```python
from build123d import *

# Parameters (mm, degrees)
BOSS_EXTRUDE1_DEPTH = 7.9
SKETCH2_R           = 1.5
CUT_EXTRUDE1_DEPTH  = 52.15085532
CUT_EXTRUDE3_DEPTH  = 3
BOSS_EXTRUDE2_DEPTH = 3
BOSS_EXTRUDE3_START = -7.9
BOSS_EXTRUDE3_DEPTH = 3
SKETCH5_W           = 8.304797865
SKETCH5_H           = 8.5
CUT_EXTRUDE4_DEPTH  = 49.987855638


with BuildPart() as part:
    # Sketch1 → Boss-Extrude1 (new body)
    with BuildSketch(Plane.XY):
        Polygon((30, 8), (30, 0), (22, 0), (22, -7), (33.5, -7), (45, 4.5), (45, 16), (38, 16), (38, 8), align=None)
    extrude(amount=-BOSS_EXTRUDE1_DEPTH)

    # Sketch2 → Cut-Extrude1 (cut, through all)
    with BuildSketch(Plane.XZ.offset(7)):
        with Locations((27, -3.95)):
            Circle(SKETCH2_R)
    cut_extrude1 = extrude(amount=-CUT_EXTRUDE1_DEPTH, mode=Mode.SUBTRACT)

    # Sketch3 → Cut-Extrude3 (cut)
    with BuildSketch(Plane(origin=(38, -7, 0), x_dir=(0, 0, -1), z_dir=(0, 1, 0))):
        Polygon((0.95, 12.732050808), (3.95, 14.464101615), (6.95, 12.732050808), (6.95, 9.267949192), (3.95, 7.535898385), (0.95, 9.267949192), align=None)
    cut_extrude3 = extrude(amount=CUT_EXTRUDE3_DEPTH, mode=Mode.SUBTRACT)

    # Sketch4 → Boss-Extrude2 (add)
    with BuildSketch(Plane.XY):
        Polygon((22, 0), (38, 16), (45, 16), (45, 4.5), (33.5, -7), (22, -7), align=None)
    extrude(amount=BOSS_EXTRUDE2_DEPTH)

    # Sketch4<3> → Boss-Extrude3 (add)
    with BuildSketch(Plane.XY.offset(BOSS_EXTRUDE3_START)):
        Polygon((30, 8), (22, 0), (30, 0), align=None)
        Polygon((30, 0), (22, 0), (22, -7), (33.5, -7), (45, 4.5), (45, 16), (38, 16), (38, 8), (30, 8), align=None)
        Polygon((38, 16), (30, 8), (38, 8), align=None)
    extrude(amount=-BOSS_EXTRUDE3_DEPTH)

    # Sketch5 → Cut-Extrude4 (cut, through all)
    with BuildSketch(Plane(origin=(0, 0, 0), x_dir=(1, 0, 0), z_dir=(0, 1, 0))):
        with Locations((26.152398932, 3.95)):
            Rectangle(SKETCH5_W, SKETCH5_H)
    cut_extrude4 = extrude(amount=CUT_EXTRUDE4_DEPTH, mode=Mode.SUBTRACT)

    # Mirror1: Cut-Extrude1, Cut-Extrude3, Cut-Extrude4 across plane
    add(cut_extrude1.mirror(Plane(origin=(19, 19, 0), x_dir=(0, 0, 1), z_dir=(0.707106781186547, 0.707106781186548, 0))), mode=Mode.SUBTRACT)
    add(cut_extrude3.mirror(Plane(origin=(19, 19, 0), x_dir=(0, 0, 1), z_dir=(0.707106781186547, 0.707106781186548, 0))), mode=Mode.SUBTRACT)
    add(cut_extrude4.mirror(Plane(origin=(19, 19, 0), x_dir=(0, 0, 1), z_dir=(0.707106781186547, 0.707106781186548, 0))), mode=Mode.SUBTRACT)


solid = part.part
```
Design review of the part built by this model. Coordinates are the model's own, in mm. A direction names the side the tool comes from. Give positions to 0.01 mm unless a question says otherwise; leave off trailing zeros. Order: outer loops, then holes, each group sorted by start corner. A loop starts at its lowest first (then second) coordinate and runs counter-clockwise, first axis right, second up. Notation, with made-up numbers: (9.5, 56) - (15.5, 56) arc R20 ccw to (15.5, 79) - close; hole circle Ø10 at (42.25, 42.5). An arc over 180 degrees is marked (long way). Use a Markdown table: item, result. Add a question column.
(1) Add section B-B on y = 11. Give the boundary of the cut face in (x, z), then the cut area to 3 significant figures.
(2) Wall thickness on probe 1 along Z at (x, y) = (27, -1.8); probe 2 along Z at (x, y) = (32, 8.5); probe 3 along Y at (x, z) = (23.5, -1): over which ranges is each line inside the solid? List them lowest first. Write a range as [from, to].
(3) Clearance check with flat-ended pins moving along their axes: P1, Ø4, axis at x = 26, y = 8.5, coming from the +Z side; P2, Ø4, axis at x = 25, z = -4, coming from the +Y side; P3, Ø3.5, axis at y = 11, z = -3.95, coming from the -X side; P4, Ø6, axis at y = 10.5, z = -8.5, coming from the -X side. State where each tip first meets the part, or that it passes through.
(4) Add section C-C on z = -4.75. Give the boundary of the cut face in (x, y).
(5) Mouldability with a two-part tool opening along X and no side actions: class faces 6 (the face through (30, 8, 2)), 7 (the face through (43.521, 8.414, -5.471)), 8 (the face through (39.2, -1.3, -3.9)), 9 (the face through (27, -6, -6.95)) as +X half, -X half, draft (parallel to the pull), parting line (faces both ways), or undercut.
(6) Machinability: for faces 1 (the face through (34, 7.695, -4)), 2 (the face through (22, -3, -4)), 3 (the face through (28.5, -4, -4.7)), 4 (the face through (34, 5, 3)), 5 (the face through (44, 11, -6.95)), which of the approach directions +Z, -Z, +X, -X, +Y, -Y give a long, thin tool a straight path to every point of the face, cutting with its end or side? Answer none if there is none.
(7) Add section A-A on x = 27. Give the boundary of the cut face in (y, z).
(8) Add section D-D on x = 41.5. Give the boundary of the cut face in (y, z).
Report:
| question | item | result |
|---|---|---|
| 1 | outline | (33, -10.9) - (45, -10.9) - (45, -6.95) - (42, -6.95) - (42, -5.45) - (38, -5.45) - (38, -8.2) - (33, -8.2) - close; (33, 0.3) - (38, 0.3) - (38, -2.45) - (42, -2.45) - (42, -0.95) - (45, -0.95) - (45, 3) - (33, 3) - close |
| 1 | area | 94.3 mm² |
| 2 | probe 1 | z = [-10.9, -5.45], [-2.45, 3] |
| 2 | probe 2 | z = [-10.9, -8.2], [0.3, 3] |
| 2 | probe 3 | y = [-7, 0] |
| 3 | P1 | passes through |
| 3 | P2 | stops at y = 0 |
| 3 | P3 | stops at x = 38 |
| 3 | P4 | stops at x = 29.5 |
| 4 | outline | (22, -7) - (24, -7) - (24, -4) - (25.73, -4) - (25.73, 0) - (22, 0) - close; (28.27, -4) - (30, -4) - (30, -7) - (33.5, -7) - (45, 4.5) - (45, 8) - (42, 8) - (42, 9.73) - (38, 9.73) - (38, 7.7) - (30.3, 7.7) - (30.3, 0) - (28.27, 0) - close; (38, 12.27) - (42, 12.27) - (42, 14) - (45, 14) - (45, 16) - (38, 16) - close |
| 5 | face 6 | -X half |
| 5 | face 7 | draft |
| 5 | face 8 | +X half |
| 5 | face 9 | undercut |
| 6 | face 1 | -X, +Y |
| 6 | face 2 | +Z, -Z, -X, +Y, -Y |
| 6 | face 3 | -Y |
| 6 | face 4 | +Z, +X, -X, +Y, -Y |
| 6 | face 5 | +X |
| 7 | outline | (-7, -10.9) - (5, -10.9) - (5, -8.2) - (0, -8.2) - (0, -5.45) - (-4, -5.45) - (-4, -6.95) - (-7, -6.95) - close; (-7, -0.95) - (-4, -0.95) - (-4, -2.45) - (0, -2.45) - (0, 0.3) - (5, 0.3) - (5, 3) - (-7, 3) - close |
| 8 | outline | (1, -10.9) - (16, -10.9) - (16, 3) - (1, 3) - close; hole circle Ø3 at (11, -3.95) |
